Source: CAD feature listing. Evaluate the final solid. Frame: model axes, mm. Coordinates: 2 decimals unless noted, no trailing zeros. Loops run counter-clockwise (first coordinate to the right, second up) from the corner with the lowest first, then second, coordinate; pieces in that order, holes last.
Item 1: Pull-direction query (X, two-part tool) for faces 1 (the flat face through (-1, 4, -5)), 2 (the flat face through (24.998, 2, -45)), 3 (the flat face through (-24.998, 2, -45)); classes: +X half, -X half, draft (parallel to the pull), parting line (faces both ways), or undercut.
Item 2: Section query C-C, the plane z = 11. Return the cut outline in (x, y), then the cut area to 3 significant figures.
Item 3: Pin query (flat end, axial travel): pin 1 Ø6 at (x, z) = (27.5, 27.5) entering from -Y; pin 2 Ø1.2 at (y, z) = (2.5, -43.5) entering from +X; pin 3 Ø1 at (x, y) = (-31, 0.5) entering from +Z. Return the tip coordinate at first contact, or that it passes through.
Item 4: Line query: probe 1 along Z at (x, y) = (0, 1.3); probe 2 along X at (y, z) = (2.5, -44); probe 3 along X at (y, z) = (2.9, 1). Output: solid intervals per line, ascending.
Item 5: Section query B-B, the plane x = 20.5. Return the cut outline in (y, z), then the cut area to 3 significant figures.
Item 6: Section query A-A, the plane y = 1.65. Return the cut outline in (x, z), then the cut area to 3 significant figures.
```python
from build123d import *

# Parameters (mm, degrees)
SKETCH_1_R      = 0.8
EXTRUDE_1_DEPTH = 4


with BuildPart() as part:
    # 스케치1 → 보스-돌출1 (new body)
    with BuildSketch(Plane.XZ):
        with BuildLine():
            Line((-24.997908733, -39.688640814), (-24.997908733, -50.327538671))
            Line((-24.997908733, -50.327538671), (24.997908733, -49.680827096))
            Line((24.997908733, -49.680827096), (24.997908733, -39.688640814))
            ThreePointArc((24.997908733, -39.688640814), (26.289808105, -32.617080103), (29.998605822, -26.459093876))
            ThreePointArc((29.998605822, -26.459093876), (0, 40), (-29.998605822, -26.459093876))
            ThreePointArc((-29.998605822, -26.459093876), (-26.289808105, -32.617080103), (-24.997908733, -39.688640814))
        make_face()
        with Locations((37, 0)):
            Circle(SKETCH_1_R, mode=Mode.SUBTRACT)
        with Locations((0, 37)):
            Circle(SKETCH_1_R, mode=Mode.SUBTRACT)
        with Locations((-37, 0)):
            Circle(SKETCH_1_R, mode=Mode.SUBTRACT)
        with Locations((0, -47.00393191)):
            Circle(SKETCH_1_R, mode=Mode.SUBTRACT)
    extrude(amount=-EXTRUDE_1_DEPTH)


solid = part.part
```
Verdict:
1. face 1: draft
1. face 2: +X half
1. face 3: -X half
2. outline: (-38.46, 0) - (38.46, 0) - (38.46, 4) - (-38.46, 4) - close
2. area: 308 mm2
3. pin 1: stops at y = 0
3. pin 2: stops at x = 25
3. pin 3: stops at z = 25.88
4. probe 1: z = -50 to -47.8, -46.2 to 36.2, 37.8 to 40
4. probe 2: x = -25 to 25
4. probe 3: x = -39.99 to 39.99
5. outline: (0, -49.74) - (4, -49.74) - (4, 34.35) - (0, 34.35) - close
5. area: 336 mm2
6. outline: (-30, -26.46) arc R20 cw to (-25, -39.69) - (-25, -50.33) - (25, -49.68) - (25, -39.69) arc R20 cw to (30, -26.46) arc R40 ccw (long way) to start; hole circle Ø1.6 at (-37, 0); hole circle Ø1.6 at (0, -47); hole circle Ø1.6 at (0, 37); hole circle Ø1.6 at (37, 0)
6. area: 5,670 mm2
